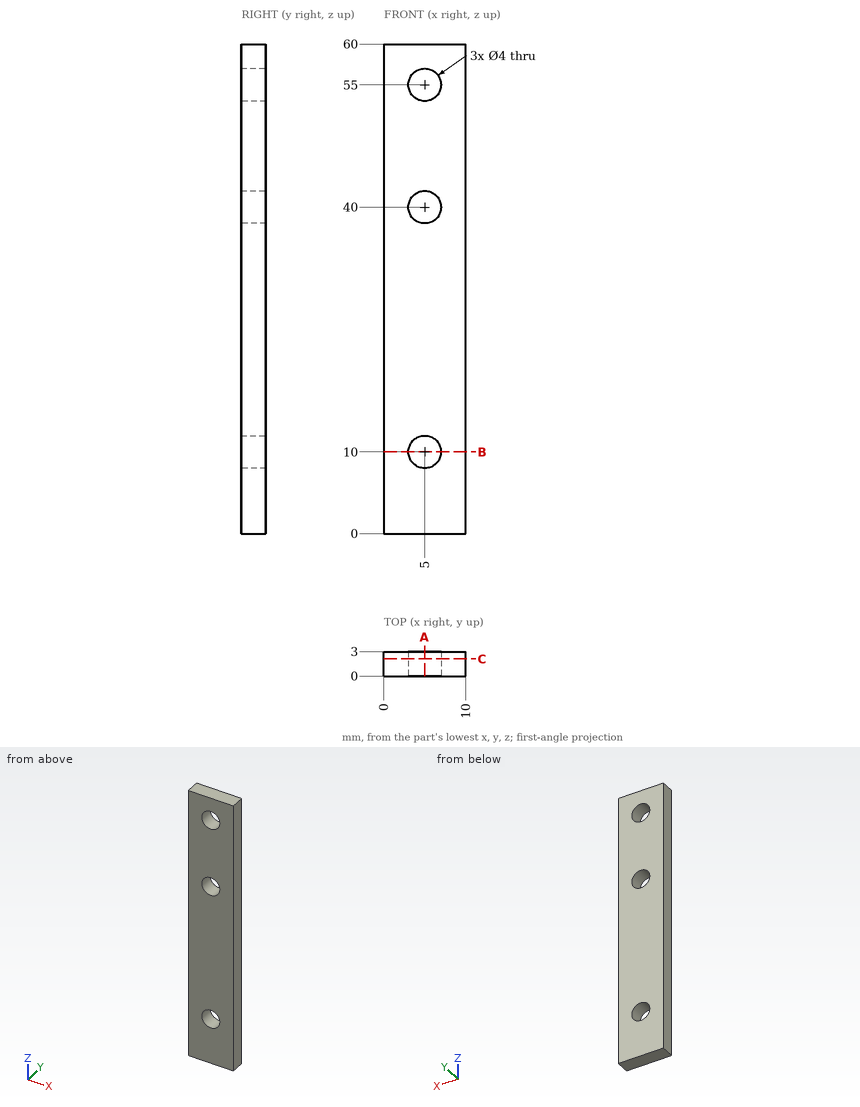
Answer from the drawing. Dimensions are ordinates in mm from the lowest x, y and z of the part. Give positions to 0.01 mm unless a question says otherwise; leave off trailing zeros. Write each loop counter-clockwise with the first axis right and the second up, starting at its lowest first coordinate (ties: lowest second). Pieces come first, ordered by that corner, then holes. Notation, with made-up numbers: (-15, -17) - (3, -17) arc R19 cw to (3, 11) - close; hole circle Ø5 at (54, 32.25). An arc over 180 degrees is marked (long way). Answer in a Markdown table with one row per item. Add a question column.
Item 1: Section C-C, the plane y = 2.1 is taken. Write down the section's boundary in (x, z), and give its area (3 significant figures).
Item 2: Find the intervals of material crossed by L1, parallel to X at y = 1.4, z = 10; L2, parallel to Z at x = 5.75, y = 1.6; L3, parallel to X at y = 1, z = 54, in increasing order.
Item 3: Section B-B, the plane z = 10 is taken. Write down the section's boundary in (x, y).
Item 4: Section A-A, the plane x = 5 is taken. Write down the section's boundary in (y, z), and give its area (3 significant figures).
Recorded:
| question | item | result |
|---|---|---|
| 1 | outline | (0, 0) - (10, 0) - (10, 60) - (0, 60) - close; hole circle Ø4 at (5, 10); hole circle Ø4 at (5, 40); hole circle Ø4 at (5, 55) |
| 1 | area | 562 mm2 |
| 2 | L1 | x = 0 to 3, 7 to 10 |
| 2 | L2 | z = 0 to 8.15, 11.85 to 38.15, 41.85 to 53.15, 56.85 to 60 |
| 2 | L3 | x = 0 to 3.27, 6.73 to 10 |
| 3 | outline | (0, 0) - (3, 0) - (3, 3) - (0, 3) - close; (7, 0) - (10, 0) - (10, 3) - (7, 3) - close |
| 4 | outline | (0, 0) - (3, 0) - (3, 8) - (0, 8) - close; (0, 12) - (3, 12) - (3, 38) - (0, 38) - close; (0, 42) - (3, 42) - (3, 53) - (0, 53) - close; (0, 57) - (3, 57) - (3, 60) - (0, 60) - close |
| 4 | area | 144 mm2 |
